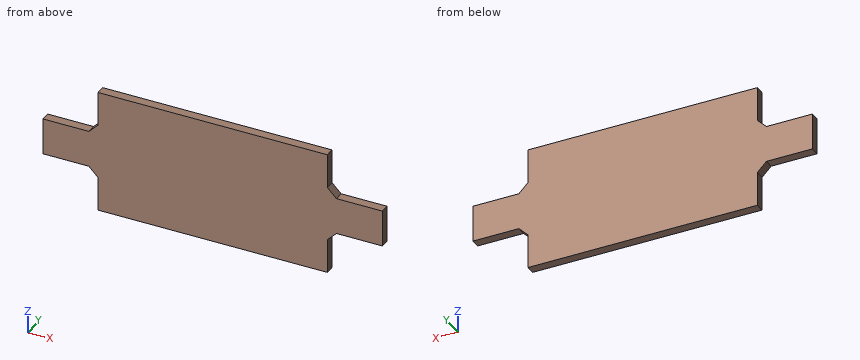
from build123d import *

# Parameters (mm, degrees)
BOSS_EXTRUDE1_DEPTH = 10
CHAMFER1_SIZE       = 10


with BuildPart() as part:
    # Sketch1 → Boss-Extrude1 (new body)
    with BuildSketch(Plane(origin=(0, 0, 0), x_dir=(1, 0, 0), z_dir=(0, 1, 0))):
        Polygon((125, -20), (125, -67.5), (-125, -67.5), (-125, -20), (-185, -20), (-185, 20), (-125, 20), (-125, 67.5), (125, 67.5), (125, 20), (185, 20), (185, -20), align=None)
    extrude(amount=BOSS_EXTRUDE1_DEPTH)

    # Chamfer1
    chamfer1_edges = [part.edges().sort_by_distance(p)[0] for p in [
        (-125, 5, 20),
        (-125, 5, -20),
        (125, 5, -20),
        (125, 5, 20),
    ]]
    chamfer(chamfer1_edges, length=CHAMFER1_SIZE)


solid = part.part
The model under review builds one solid part; all positions refer to its coordinate system, in mm. Coordinates: 2 decimals unless noted, no trailing zeros. Loops run counter-clockwise (first coordinate to the right, second up) from the corner with the lowest first, then second, coordinate; pieces in that order, holes last. Notation, with made-up numbers: M -21,-7.5 L -15,-7.5 A18 ccw -15,21.5 Z; hole C 63,72 d3. An arc over 180 degrees is marked long. Put each result on its own line as item: value. Start each with the question number.
Q1. Add section A-A (y = 7.5). Write out the cut boundary in (x, z), and give its area (4 significant figures).
Q2. Wall thickness on line 1 (X direction, y = 5.5, z = -37.5); line 2 (Z direction, x = -166, y = 3); line 3 (X direction, y = 4, z = -27): over which ranges is each line inside the solid? List them lowest first.
Q3. Add section C-C (x = 130.5). Write out the cut boundary in (y, z), and give its area (3 significant figures).
Q4. Clearance check with flat-ended pins moving along their axes: pin 1 (5 mm diameter, centred on y = 5, z = 52, fed in from -X); pin 2 (3 mm diameter, centred on x = -170.5, y = 3, fed in from -Z); pin 3 (5 mm diameter, centred on y = 4, z = -41, fed in from +X). State where each tip first meets the part, or that it passes through.
Q5. Add section B-B (z = 57). Write out the cut boundary in (x, y), and give its area (3 significant figures).
Answers:
1. outline: M -185,-20 L -135,-20 L -125,-30 L -125,-67.5 L 125,-67.5 L 125,-30 L 135,-20 L 185,-20 L 185,20 L 135,20 L 125,30 L 125,67.5 L -125,67.5 L -125,30 L -135,20 L -185,20 Z
1. area: 38,750 mm^2
2. line 1: x = -125 to 125
2. line 2: z = -20 to 20
2. line 3: x = -128 to 128
3. outline: M 0,-24.5 L 10,-24.5 L 10,24.5 L 0,24.5 Z
3. area: 490 mm^2
4. pin 1: stops at x = -125
4. pin 2: stops at z = -20
4. pin 3: stops at x = 125
5. outline: M -125,0 L 125,0 L 125,10 L -125,10 Z
5. area: 2,500 mm^2
